The figure shows three views and two pictorial views of one solid part (mm, origin at its lowest corner). Answer the questions. A direction names the side the tool comes from. Coordinates: 2 decimals unless noted, no trailing zeros. Order: outer loops, then holes, each group sorted by start corner. A loop starts at its lowest first (then second) coordinate and runs counter-clockwise, first axis right, second up. Notation, with made-up numbers: (83, -16.5) -> (106, -16.5) arc R16 ccw to (106, 0.5) -> close; hole circle Ø8 at (71.5, 5). An arc over 180 degrees is marked (long way). Return JSON: item names as keys, results as strings.
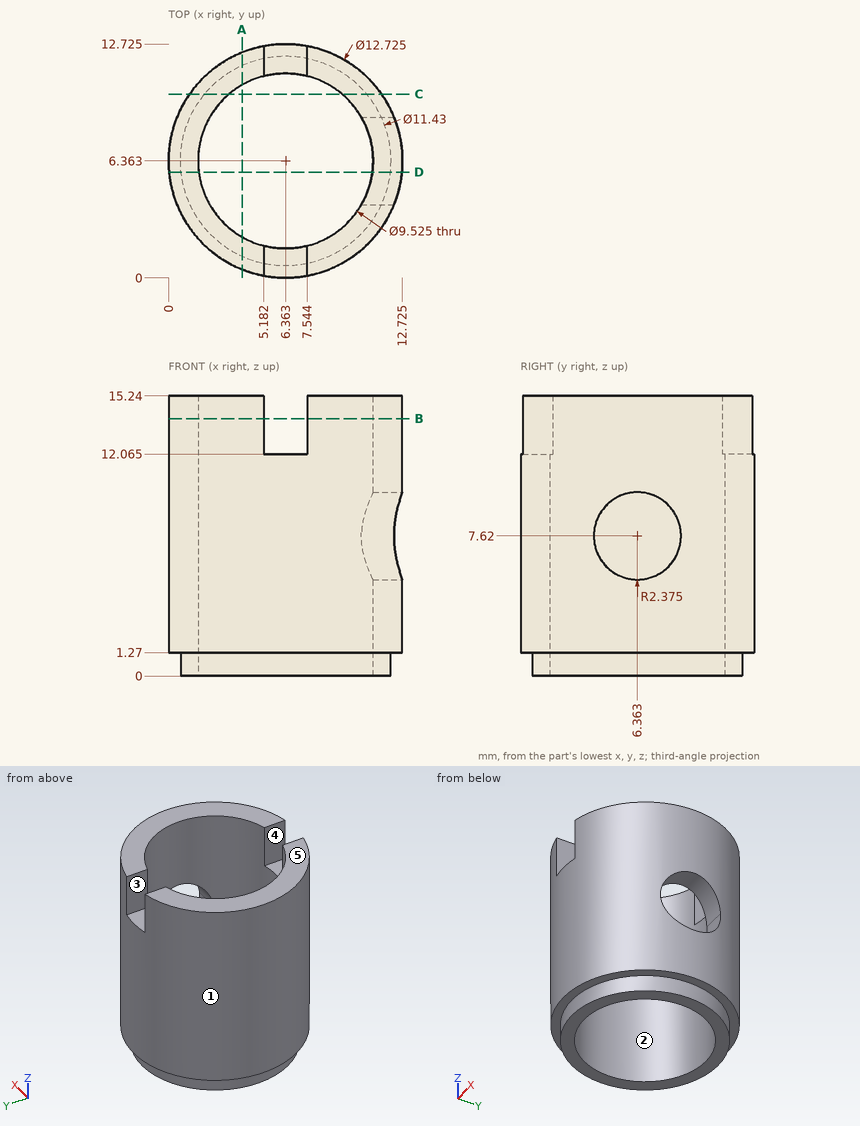
Item 1: The part is cut by section D-D on y = 5.75. Determine the outline of the cut face in (x, z) (1 decimal).
Answer list:
{"outline": "(0, 1.3) -> (0.7, 1.3) -> (0.7, 0) -> (1.6, 0) -> (1.6, 15.2) -> (0, 15.2) -> close; (11.1, 0) -> (12, 0) -> (12, 1.3) -> (12.7, 1.3) -> (12.7, 5.3) -> (11.1, 5.3) -> close; (11.1, 9.9) -> (12.7, 9.9) -> (12.7, 15.2) -> (11.1, 15.2) -> close"}
Item 2: The part is cut by section C-C on y = 10. Determine the outline of the cut face in (x, z) (1 decimal).
Answer list:
{"outline": "(1.1, 1.3) -> (2, 1.3) -> (2, 0) -> (3.3, 0) -> (3.3, 15.2) -> (1.1, 15.2) -> close; (9.4, 0) -> (10.8, 0) -> (10.8, 1.3) -> (11.6, 1.3) -> (11.6, 15.2) -> (9.4, 15.2) -> close"}
Item 3: Which of the six approach directions +Z, -Z, +X, -X, +Y, -Y give full straight-line access (tool end or side, diameter ignored) to the marked faces 4 and 5?
Answer list:
{"face 4": "+Z, +Y, -Y", "face 5": "+Z, +X, -X, +Y, -Y"}
Item 4: The part is cut by section A-A on x = 4. Determine the outline of the cut face in (y, z) (1 decimal).
Answer list:
{"outline": "(0.5, 1.3) -> (1.2, 1.3) -> (1.2, 0) -> (2.2, 0) -> (2.2, 15.2) -> (0.5, 15.2) -> close; (10.5, 0) -> (11.6, 0) -> (11.6, 1.3) -> (12.3, 1.3) -> (12.3, 15.2) -> (10.5, 15.2) -> close"}
Item 5: The part is cut by section B-B on z = 14. Determine the outline of the cut face in (x, y) (1 decimal).
Answer list:
{"outline": "(5.2, 0.1) -> (5.2, 1.7) arc R4.8 cw to (5.2, 11) -> (5.2, 12.6) arc R6.4 ccw to start; (7.5, 0.1) arc R6.4 ccw to (7.5, 12.6) -> (7.5, 11) arc R4.8 cw to (7.5, 1.7) -> close"}
Item 6: Flat-ended cylindrical pins translate along their axes: pin 1 (1.8 mm diameter, centred on y = 1.5, z = 13.5, fed in from -X) (1 decimal); pin 2 (0.5 mm diameter, centred on x = 7, y = 1.5, fed in from +Z) (3 decimals); pin 3 (1 mm diameter, centred on x = 2.5, z = 10, fed in from -Y); pin 4 (6.5 mm diameter, centred on x = 7, y = 7.5, fed in from -Z) (3 decimals). Find the tip coordinate at first contact, or state that the pin passes through.
Answer list:
{"pin 1": "x = 1.4", "pin 2": "z = 12.065", "pin 3": "y = 0.96", "pin 4": "through"}
Item 7: Find the intervals of material crossed by probe 1 along Y at (x, z) = (6.5, 8.5); probe 2 along Z at (x, y) = (2.75, 11.5); probe 3 along X at (y, z) = (8.5, 3) (1 decimal), in increasing order.
Answer list:
{"probe 1": "0 to 1.6, 11.12 to 12.72", "probe 2": "1.27 to 15.24", "probe 3": "0.4 to 2.1, 10.6 to 12.4"}
Item 8: Determine the mould class of the marked faces 1, 2 and 3 for opening direction Y: pulls with the +Y half, pulls with the -Y half, needs draft (parallel to the pull), parting line crosses it, or undercut.
Answer list:
{"face 1": "parting line crosses it", "face 2": "undercut", "face 3": "needs draft"}
